from build123d import *

# Parameters (mm, degrees)
SKETCH3_W           = 63.5
SKETCH3_H           = 88.9
BOSS_EXTRUDE1_DEPTH = 2.54
BOSS_EXTRUDE2_DEPTH = 25.4
SKETCH5_R           = 3.01625
BOSS_EXTRUDE3_DEPTH = 5.08
FILLET1_R           = 2.54
FILLET2_R           = 2.54
SKETCH6_W           = 12.7
SKETCH6_H           = 3.175
BOSS_EXTRUDE4_DEPTH = 6.35
CUT_EXTRUDE1_REACH  = 80.878
SKETCH7_R           = 1.4732
SKETCH8_W           = 12.7
SKETCH8_H           = 3.175
BOSS_EXTRUDE5_DEPTH = 11.43
CUT_EXTRUDE2_REACH  = 80.878
SKETCH9_R           = 1.4732


with BuildPart() as part:
    # Sketch3 → Boss-Extrude1 (new body)
    with BuildSketch(Plane(origin=(0, 0, 0), x_dir=(1, 0, 0), z_dir=(0, 1, 0))):
        Rectangle(SKETCH3_W, SKETCH3_H)
    extrude(amount=BOSS_EXTRUDE1_DEPTH)

    # Sketch4 → Boss-Extrude2 (add)
    with BuildSketch(Plane(origin=(0, 0, 0), x_dir=(1, 0, 0), z_dir=(0, 1, 0))):
        Polygon((-31.75, -44.45), (-31.75, 44.45), (31.75, 44.45), (31.75, -44.45), (31.75, -49.53), (36.83, -49.53), (36.83, 49.53), (-36.83, 49.53), (-36.83, -49.53), (-31.75, -49.53), align=None)
    extrude(amount=BOSS_EXTRUDE2_DEPTH)

    # Sketch5 → Boss-Extrude3 (add)
    with BuildSketch(Plane.ZY.offset(36.83)):
        with BuildLine():
            Line((-46.99, 34.29), (-46.99, 0))
            Line((-46.99, 0), (-33.3375, 0))
            Line((-33.3375, 0), (-33.3375, 34.29))
            ThreePointArc((-33.3375, 34.29), (-40.16375, 41.11625), (-46.99, 34.29))
        make_face()
        with Locations((-40.16375, 34.29)):
            Circle(SKETCH5_R, mode=Mode.SUBTRACT)
    boss_extrude3 = extrude(amount=BOSS_EXTRUDE3_DEPTH)

    # Mirror1: Boss-Extrude3 across plane
    add(boss_extrude3.mirror(Plane(origin=(0, 0, 0), x_dir=(0, 0, 1), z_dir=(1, 0, 0))))

    # Fillet1
    fillet1_edges = [part.edges().sort_by_distance(p)[0] for p in [
        (-36.83, 12.7, -46.99),
        (-36.83, 12.7, -33.3375),
        (36.83, 12.7, -46.99),
        (36.83, 12.7, -33.3375),
    ]]
    fillet(fillet1_edges, radius=FILLET1_R - 0.0001)  # a hair under: the kernel refuses the full size

    # Fillet2
    fillet2_edges = [part.edges().sort_by_distance(p)[0] for p in [
        (38.09995, 25.4, -33.3375),
        (36.83, 25.4, -40.16375),
        (38.09995, 25.4, -46.99),
        (-38.09995, 25.4, -46.99),
        (-36.83, 25.4, -40.16375),
        (-38.09995, 25.4, -33.3375),
    ]]
    fillet(fillet2_edges, radius=FILLET2_R - 0.0004)  # a hair under: the kernel refuses the full size

    # Sketch6 → Boss-Extrude4 (add)
    with BuildSketch(Plane.ZY.offset(41.91)):
        with Locations((-40.16375, 1.5875)):
            Rectangle(SKETCH6_W, SKETCH6_H)
    boss_extrude4 = extrude(amount=BOSS_EXTRUDE4_DEPTH)

    # Sketch7 → Cut-Extrude1 (cut, up to next)
    with BuildSketch(Plane(origin=(0, 3.175, 0), x_dir=(1, 0, 0), z_dir=(0, 1, 0)), mode=Mode.PRIVATE) as cut_extrude1_sk1:
        with Locations(Location((-45.085, 40.16375, 0), (0, 0, 270))):
            Circle(SKETCH7_R)
    cut_extrude1_tool1 = extrude(cut_extrude1_sk1.sketch, amount=-CUT_EXTRUDE1_REACH, mode=Mode.PRIVATE) & part.part
    cut_extrude1 = cut_extrude1_tool1.solids().sort_by_distance((-45.085, 3.175, -40.16375))[0]
    add(cut_extrude1, mode=Mode.SUBTRACT)

    # Sketch8 → Boss-Extrude5 (add)
    with BuildSketch(Plane.ZY.offset(36.83)):
        with Locations((38.1, 1.5875)):
            Rectangle(SKETCH8_W, SKETCH8_H)
    boss_extrude5 = extrude(amount=BOSS_EXTRUDE5_DEPTH)

    # Sketch9 → Cut-Extrude2 (cut, up to next)
    with BuildSketch(Plane(origin=(0, 3.175, 0), x_dir=(1, 0, 0), z_dir=(0, 1, 0)), mode=Mode.PRIVATE) as cut_extrude2_sk1:
        with Locations(Location((-45.085, -38.1, 0), (0, 0, 270))):
            Circle(SKETCH9_R)
    cut_extrude2_tool1 = extrude(cut_extrude2_sk1.sketch, amount=-CUT_EXTRUDE2_REACH, mode=Mode.PRIVATE) & part.part
    cut_extrude2 = cut_extrude2_tool1.solids().sort_by_distance((-45.085, 3.175, 38.1))[0]
    add(cut_extrude2, mode=Mode.SUBTRACT)

    # Mirror2: Boss-Extrude4, Cut-Extrude1, Boss-Extrude5, Cut-Extrude2 across plane
    add(boss_extrude4.mirror(Plane(origin=(0, 0, 0), x_dir=(0, 0, 1), z_dir=(1, 0, 0))))
    add(cut_extrude1.mirror(Plane(origin=(0, 0, 0), x_dir=(0, 0, 1), z_dir=(1, 0, 0))), mode=Mode.SUBTRACT)
    add(boss_extrude5.mirror(Plane(origin=(0, 0, 0), x_dir=(0, 0, 1), z_dir=(1, 0, 0))))
    add(cut_extrude2.mirror(Plane(origin=(0, 0, 0), x_dir=(0, 0, 1), z_dir=(1, 0, 0))), mode=Mode.SUBTRACT)


solid = part.part
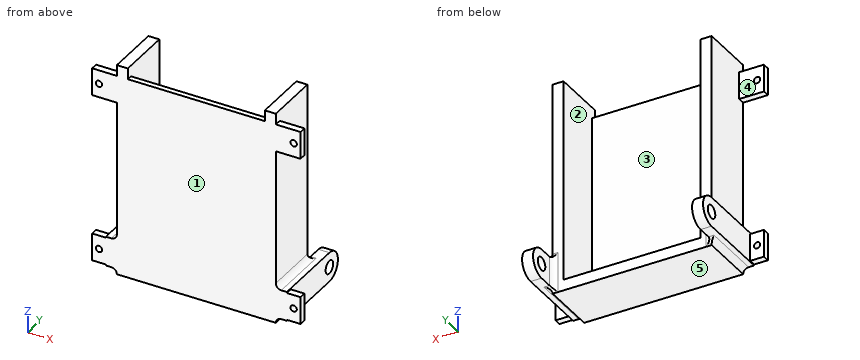
Could you check a few things on this model? Use its own coordinates, in mm. Face numbers are marked on the shaded views. A direction names the side the tool comes from. Give positions to 0.01 mm unless a question says otherwise; leave off trailing zeros. Order: outer loops, then holes, each group sorted by start corner. A loop starts at its lowest first (then second) coordinate and runs counter-clockwise, first axis right, second up.
Item 1: If we section it at A-A, the plane z = 38.1: Write out the boundary of the cut face in (x, y) (3 decimals).
Item 2: For the marked faces 3, 4 and 5, which set-ups out of +Z, -Z, +X, -X, +Y, -Y let a thin tool reach every point of the face, with its end or its side?
Item 3: I'm going to push flat-ended pins straight in: pin 1 (6 mm diameter, centred on y = 8, z = 35, fed in from -X); pin 2 (4 mm diameter, centred on y = 6.5, z = 27.5, fed in from +X); pin 3 (7 mm diameter, centred on x = -46.5, z = -37, fed in from +Y) (3 decimals); pin 4 (2.5 mm diameter, centred on x = -45.08, z = -40.16, fed in from +Y). Where does each tip first touch, or does it pass through?
Item 4: I need wall thicknesses on line 1 (X direction, y = 1.25, z = 38.1); line 2 (X direction, y = 15.5, z = -33.5); line 3 (X direction, y = 39, z = -39). Which ranges of each line are inside material? Lowest first, please.
Item 5: If we mould it in two halves opening along X, with no side actions, what happens to the marked faces 1 and 2? For each: pulls with the +X half, pulls with the -X half, needs draft (parallel to the pull), parting line crosses it, or undercut.
Item 6: If we section it at C-C, the plane x = 28: Write out the boundary of the cut face in (y, z), plus the area to 3 significant figures.
Item 7: If we section it at D-D, the plane z = 20: Write out the boundary of the cut face in (x, y).
Values:
1. outline: (-48.26, 0) - (-46.558, 0) - (-46.558, 3.175) - (-48.26, 3.175) - close; (-43.612, 0) - (43.612, 0) - (43.612, 3.175) - (36.83, 3.175) - (36.83, 25.4) - (31.75, 25.4) - (31.75, 2.54) - (-31.75, 2.54) - (-31.75, 25.4) - (-36.83, 25.4) - (-36.83, 3.175) - (-43.612, 3.175) - close; (46.558, 0) - (48.26, 0) - (48.26, 3.175) - (46.558, 3.175) - close
2. face 3: +Z, +Y
2. face 4: +Z, -X, +Y
2. face 5: -Z, +X, -X, +Y, -Y
3. pin 1: stops at x = -36.83
3. pin 2: stops at x = 36.83
3. pin 3: stops at y = 3.175
3. pin 4: passes through
4. line 1: x = -48.26 to -46.56, -43.61 to 43.61, 46.56 to 48.26
4. line 2: x = -41.91 to -31.75, 31.75 to 41.91
4. line 3: x = -41.91 to -36.83, 36.83 to 41.91
5. face 1: needs draft
5. face 2: undercut
6. outline: (0, -49.53) - (25.4, -49.53) - (25.4, -44.45) - (2.54, -44.45) - (2.54, 44.45) - (0, 44.45) - close
6. area: 355 mm2
7. outline: (-36.83, 0) - (36.83, 0) - (36.83, 25.4) - (31.75, 25.4) - (31.75, 2.54) - (-31.75, 2.54) - (-31.75, 25.4) - (-36.83, 25.4) - close
